from build123d import *

# Parameters (mm, degrees)
SKIZZE1_W                       = 410
SKIZZE1_H                       = 410
AUFSATZ_LINEAR_AUSTRAGEN1_DEPTH = 5
SKIZZE2_W                       = 97.796702903
SKIZZE2_H                       = 49.6
SCHNITT_LINEAR_AUSTRAGEN1_DEPTH = 5
LINEARES_MUSTER1_COUNT          = 4
LINEARES_MUSTER1_PITCH          = 99.9
SPIEGELN1_COPY_1_SKETCH_W       = 97.796702903
SPIEGELN1_COPY_1_SKETCH_H       = 49.6
SPIEGELN1_COPY_1_DEPTH          = 5
SPIEGELN1_COPY_2_SKETCH_W       = 97.796702903
SPIEGELN1_COPY_2_SKETCH_H       = 49.6
SPIEGELN1_COPY_2_DEPTH          = 5
SPIEGELN1_COPY_3_SKETCH_W       = 97.796702903
SPIEGELN1_COPY_3_SKETCH_H       = 49.6
SPIEGELN1_COPY_3_DEPTH          = 5
SKIZZE3_W                       = 49.6
SKIZZE3_H                       = 41.77912255
SCHNITT_LINEAR_AUSTRAGEN2_DEPTH = 5
LINEARES_MUSTER2_COUNT          = 4
LINEARES_MUSTER2_PITCH          = 99.9
SPIEGELN2_COPY_1_SKETCH_W       = 49.6
SPIEGELN2_COPY_1_SKETCH_H       = 41.77912255
SPIEGELN2_COPY_1_DEPTH          = 5
SPIEGELN2_COPY_2_SKETCH_W       = 49.6
SPIEGELN2_COPY_2_SKETCH_H       = 41.77912255
SPIEGELN2_COPY_2_DEPTH          = 5
SPIEGELN2_COPY_3_SKETCH_W       = 49.6
SPIEGELN2_COPY_3_SKETCH_H       = 41.77912255
SPIEGELN2_COPY_3_DEPTH          = 5
SCHNITT_LINEAR_AUSTRAGEN3_DEPTH = 5
SPIEGELN4_COPY_1_DEPTH          = 5
SKIZZE5_R                       = 2.5
SCHNITT_LINEAR_AUSTRAGEN4_DEPTH = 10
LINEARES_MUSTER3_COUNT          = 6
LINEARES_MUSTER3_PITCH          = 12
LINEARES_MUSTER3_COUNT_DIR2     = 6
LINEARES_MUSTER3_PITCH_DIR2     = 12


with BuildPart() as part:
    # Skizze1 → Aufsatz-Linear austragen1 (new body)
    with BuildSketch(Plane.XY):
        with Locations((205, 205)):
            Rectangle(SKIZZE1_W, SKIZZE1_H)
    extrude(amount=AUFSATZ_LINEAR_AUSTRAGEN1_DEPTH)

    # Skizze2 → Schnitt-Linear austragen1 (cut)
    with BuildSketch(Plane.XY.offset(5)):
        with Locations((-43.898351452, 354.85)):
            Rectangle(SKIZZE2_W, SKIZZE2_H)
    schnitt_linear_austragen1 = extrude(amount=-SCHNITT_LINEAR_AUSTRAGEN1_DEPTH, mode=Mode.SUBTRACT)

    # Lineares Muster1: Schnitt-Linear austragen1 ×4
    with Locations(*[(0, -i * LINEARES_MUSTER1_PITCH, 0) for i in range(1, LINEARES_MUSTER1_COUNT)]):
        add(schnitt_linear_austragen1, mode=Mode.SUBTRACT)

    # Spiegeln1: Schnitt-Linear austragen1 across plane
    add(schnitt_linear_austragen1.mirror(Plane(origin=(205, 0, 0), x_dir=(0, 0, 1), z_dir=(1, 0, 0))), mode=Mode.SUBTRACT)

    # Spiegeln1 copy 1 sketch → Spiegeln1 copy 1 (cut)
    with BuildSketch(Plane(origin=(410, -99.9, 5), x_dir=(-1, 0, 0), z_dir=(0, 0, 1))):
        with Locations((-43.898351452, -354.85)):
            Rectangle(SPIEGELN1_COPY_1_SKETCH_W, SPIEGELN1_COPY_1_SKETCH_H)
    extrude(amount=-SPIEGELN1_COPY_1_DEPTH, mode=Mode.SUBTRACT)

    # Spiegeln1 copy 2 sketch → Spiegeln1 copy 2 (cut)
    with BuildSketch(Plane(origin=(410, -199.8, 5), x_dir=(-1, 0, 0), z_dir=(0, 0, 1))):
        with Locations((-43.898351452, -354.85)):
            Rectangle(SPIEGELN1_COPY_2_SKETCH_W, SPIEGELN1_COPY_2_SKETCH_H)
    extrude(amount=-SPIEGELN1_COPY_2_DEPTH, mode=Mode.SUBTRACT)

    # Spiegeln1 copy 3 sketch → Spiegeln1 copy 3 (cut)
    with BuildSketch(Plane(origin=(410, -299.7, 5), x_dir=(-1, 0, 0), z_dir=(0, 0, 1))):
        with Locations((-43.898351452, -354.85)):
            Rectangle(SPIEGELN1_COPY_3_SKETCH_W, SPIEGELN1_COPY_3_SKETCH_H)
    extrude(amount=-SPIEGELN1_COPY_3_DEPTH, mode=Mode.SUBTRACT)

    # Skizze3 → Schnitt-Linear austragen2 (cut)
    with BuildSketch(Plane.XY.offset(5)):
        with Locations((55.15, 425.889561275)):
            Rectangle(SKIZZE3_W, SKIZZE3_H)
    schnitt_linear_austragen2 = extrude(amount=-SCHNITT_LINEAR_AUSTRAGEN2_DEPTH, mode=Mode.SUBTRACT)

    # Lineares Muster2: Schnitt-Linear austragen2 ×4
    with Locations(*[(i * LINEARES_MUSTER2_PITCH, 0, 0) for i in range(1, LINEARES_MUSTER2_COUNT)]):
        add(schnitt_linear_austragen2, mode=Mode.SUBTRACT)

    # Spiegeln2: Schnitt-Linear austragen2 across plane
    add(schnitt_linear_austragen2.mirror(Plane.ZX.offset(205)), mode=Mode.SUBTRACT)

    # Spiegeln2 copy 1 sketch → Spiegeln2 copy 1 (cut)
    with BuildSketch(Plane(origin=(99.9, 410, 5), x_dir=(1, 0, 0), z_dir=(0, 0, 1))):
        with Locations((55.15, -425.889561275)):
            Rectangle(SPIEGELN2_COPY_1_SKETCH_W, SPIEGELN2_COPY_1_SKETCH_H)
    extrude(amount=-SPIEGELN2_COPY_1_DEPTH, mode=Mode.SUBTRACT)

    # Spiegeln2 copy 2 sketch → Spiegeln2 copy 2 (cut)
    with BuildSketch(Plane(origin=(199.8, 410, 5), x_dir=(1, 0, 0), z_dir=(0, 0, 1))):
        with Locations((55.15, -425.889561275)):
            Rectangle(SPIEGELN2_COPY_2_SKETCH_W, SPIEGELN2_COPY_2_SKETCH_H)
    extrude(amount=-SPIEGELN2_COPY_2_DEPTH, mode=Mode.SUBTRACT)

    # Spiegeln2 copy 3 sketch → Spiegeln2 copy 3 (cut)
    with BuildSketch(Plane(origin=(299.7, 410, 5), x_dir=(1, 0, 0), z_dir=(0, 0, 1))):
        with Locations((55.15, -425.889561275)):
            Rectangle(SPIEGELN2_COPY_3_SKETCH_W, SPIEGELN2_COPY_3_SKETCH_H)
    extrude(amount=-SPIEGELN2_COPY_3_DEPTH, mode=Mode.SUBTRACT)

    # Skizze4 → Schnitt-Linear austragen3 (cut)
    with BuildSketch(Plane.XY.offset(5)):
        Polygon((5, 379.65), (5, 405), (30.35, 405), (30.35, 431.549801047), (5, 431.549801047), (-47.862925009, 431.549801047), (-47.862925009, 405), (-47.862925009, 379.65), align=None)
    schnitt_linear_austragen3 = extrude(amount=-SCHNITT_LINEAR_AUSTRAGEN3_DEPTH, mode=Mode.SUBTRACT)

    # Spiegeln3: Schnitt-Linear austragen3 across plane
    add(schnitt_linear_austragen3.mirror(Plane(origin=(205, 0, 0), x_dir=(0, 0, 1), z_dir=(1, 0, 0))), mode=Mode.SUBTRACT)

    # Spiegeln4: Schnitt-Linear austragen3 across plane
    add(schnitt_linear_austragen3.mirror(Plane.ZX.offset(205)), mode=Mode.SUBTRACT)

    # Spiegeln4 copy 1 sketch → Spiegeln4 copy 1 (cut)
    with BuildSketch(Plane(origin=(410, 410, 5), x_dir=(-1, 0, 0), z_dir=(0, 0, 1))):
        Polygon((5, 379.65), (5, 405), (30.35, 405), (30.35, 431.549801047), (5, 431.549801047), (-47.862925009, 431.549801047), (-47.862925009, 405), (-47.862925009, 379.65), align=None)
    extrude(amount=-SPIEGELN4_COPY_1_DEPTH, mode=Mode.SUBTRACT)

    # Skizze5 → Schnitt-Linear austragen4 (cut)
    with BuildSketch(Plane.XY.offset(5)):
        with Locations((125, 285)):
            Circle(SKIZZE5_R)
    schnitt_linear_austragen4 = extrude(amount=-SCHNITT_LINEAR_AUSTRAGEN4_DEPTH, mode=Mode.SUBTRACT)

    # Lineares Muster3: Schnitt-Linear austragen4 6 × 6
    with Locations(*[(-j * LINEARES_MUSTER3_PITCH_DIR2, i * LINEARES_MUSTER3_PITCH, 0) for i in range(LINEARES_MUSTER3_COUNT) for j in range(LINEARES_MUSTER3_COUNT_DIR2) if (i, j) != (0, 0)]):
        add(schnitt_linear_austragen4, mode=Mode.SUBTRACT)


solid = part.part
Geometry check sheet. Reference: the model listing, model coordinates, mm. Round coordinates to 2 decimals unless told otherwise and drop trailing zeros. Order: outer loops, then holes, each group sorted by start corner. A loop starts at its lowest first (then second) coordinate and runs counter-clockwise, first axis right, second up. Notation, with made-up numbers: M -0.75,-20 L 20.25,-20 A24 cw 20.25,10 Z; hole C 57,16.25 d10. An arc over 180 degrees is marked long. Answer in a Markdown table with one row per item. Add a question column.
Item 1: Material ranges on L1, parallel to X at y = 355, z = 2.3, recorded low to high. Write a range as [from, to].
Item 2: Depth check by flat-ended pin: pin 1 Ø4 at (x, y) = (101, 345) entering from +Z; pin 2 Ø2.5 at (y, z) = (163.5, 1.5) entering from -X; pin 3 Ø1.5 at (x, z) = (54.5, 2) entering from +Y; pin 4 Ø1.5 at (y, z) = (406.5, 1.5) entering from -X. Enter the tip coordinate at first touch or a pass-through.
Item 3: Sectioned sample at B-B, the plane x = 270.5. Enter the section's corners in (y, z), plus the area to 3 significant figures.
Item 4: Sectioned sample at A-A, the plane z = 3.05. State how many separate pieces and enclosed holes the cut face has, plus the area to 3 significant figures.
Filled in:
| question | item | result |
|---|---|---|
| 1 | L1 | x = [5, 405] |
| 2 | pin 1 | passes through |
| 2 | pin 2 | stops at x = 5 |
| 2 | pin 3 | stops at y = 405 |
| 2 | pin 4 | stops at x = 79.95 |
| 3 | outline | M 5,0 L 405,0 L 405,5 L 5,5 Z |
| 3 | area | 2,000 mm² |
| 4 | separate pieces | 1 |
| 4 | enclosed holes | 36 |
| 4 | area | 162,000 mm² |
